from build123d import *

# Parameters (mm, degrees)
F0_W     = 3.81
F0_H     = 16.51
F1_DEPTH = 25.4
F2_W     = 12.7
F2_H     = 5.08
F3_DEPTH = 13.97
F4_R     = 5.08
F6_DEPTH = 25.4
F7_R     = 1.905
F8_DEPTH = 25.4


with BuildPart() as f1:
    # F0 (on Right) → F1 (new body)
    with BuildSketch(Plane.YZ):
        with Locations((-1.905, -8.255)):
            Rectangle(F0_W, F0_H)
    extrude(amount=F1_DEPTH)

    # F2 (on face) → F3 (join)
    with BuildSketch(Plane.XZ.offset(3.81)):
        Polygon((19.05, 0), (12.7, 0), (6.35, 0), (6.35, -5.08), (19.05, -5.08), align=None)
        with Locations((12.7, -13.97)):
            Rectangle(F2_W, F2_H)
    extrude(amount=F3_DEPTH)

    # F4
    f4_edges = [f1.edges().sort_by_distance(p)[0] for p in [
        (19.05, -17.78, -2.54),
        (6.35, -17.78, -2.54),
        (19.05, -17.78, -13.97),
        (6.35, -17.78, -13.97),
    ]]
    fillet(f4_edges, radius=F4_R)

    # F5 (on face) → F6 (cut)
    with BuildSketch(Plane.XY):
        with BuildLine():
            ThreePointArc((15.0495, -11.43), (11.038653, -9.768653), (12.7, -13.7795))
            ThreePointArc((12.7, -13.7795), (14.361347, -13.091347), (15.0495, -11.43))
        make_face()
    extrude(amount=-F6_DEPTH, mode=Mode.SUBTRACT)

    # F7 (on face) → F8 (cut)
    with BuildSketch(Plane.XZ.offset(3.81)):
        with Locations((3.407462, -8.255)):
            Circle(F7_R)
        with Locations((21.952828, -8.255)):
            Circle(F7_R)
    extrude(amount=-F8_DEPTH, mode=Mode.SUBTRACT)


solid = f1.part
The listing builds one solid part. Answer for the finished solid, in the listing's coordinates (mm). A direction names the side the tool comes from. Give positions to 0.01 mm unless a question says otherwise; leave off trailing zeros. Order: outer loops, then holes, each group sorted by start corner. A loop starts at its lowest first (then second) coordinate and runs counter-clockwise, first axis right, second up. Notation, with made-up numbers: (-4.75, -40) - (36.25, -40) arc R25 ccw to (36.25, -9) - close; hole circle Ø6 at (-19, 73.5). An arc over 180 degrees is marked (long way). One line per item, written item: value. Start each with the question number.
1) A cutting plane is placed at A-A on y = -4.5. Give the vertices of the cut face in (x, z).
2) A cutting plane is placed at D-D on x = 22.5. Give the vertices of the cut face in (y, z), then the cut area to 3 significant figures.
3) A cutting plane is placed at C-C on y = -13.25. Give the vertices of the cut face in (x, z).
4) Given pin 1 Ø5 at (x, z) = (11, -8.5) entering from -Y; pin 2 Ø1 at (x, y) = (4.5, -13) entering from -Z; pin 3 Ø1.5 at (y, z) = (-9.5, -13) entering from -X; pin 4 Ø1.5 at (y, z) = (-10, -2) entering from +X, each flat-ended and moving along its own axis, determine where each tip first touches the part or whether it passes through.
5) Find the intervals of material crossed by L1, parallel to X at y = -11.43, z = -3.85; L2, parallel to Z at x = 10.5, y = -6.25, in increasing order.
6) The mould has two halves that part along X. Classify faces 6 (the face through (20.05, -1.93, -8.17)), 7 (the face through (25.4, -2, -8)), 8 (the face through (13, -7, -16.51)): released by +X, released by -X, zero draft, split by the parting line, or undercut.
7) A cutting plane is placed at B-B on z = -1.75. Give the vertices of the cut face in (x, y), then the cut area to 3 significant figures.
8) A tool of negligible diameter and unlimited length cuts with its end or side. For faces 1 (the face through (13, -17.78, -14)), 2 (the face through (19.05, -8, -3)), 3 (the face through (6.35, -8, -14)), 4 (the face through (13, 0, -8)), 5 (the face through (14, -9, -5.08)), from which of +Z, -Z, +X, -X, +Y, -Y can it reach the whole face along a straight path? Write none if from no direction.
Answer sheet:
1. outline: (6.35, -16.51) - (19.05, -16.51) - (19.05, -11.43) - (6.35, -11.43) - close; (6.35, -5.08) - (19.05, -5.08) - (19.05, 0) - (6.35, 0) - close
2. outline: (-3.81, -16.51) - (0, -16.51) - (0, -10.08) - (-3.81, -10.08) - close; (-3.81, -6.43) - (0, -6.43) - (0, 0) - (-3.81, 0) - close
2. area: 49.0 mm2
3. outline: (6.38, -16.51) - (11.21, -16.51) - (11.21, -11.43) - (6.38, -11.43) - close; (6.38, -5.08) - (11.21, -5.08) - (11.21, 0) - (6.38, 0) - close; (14.19, -16.51) - (19.02, -16.51) - (19.02, -11.43) - (14.19, -11.43) - close; (14.19, -5.08) - (19.02, -5.08) - (19.02, 0) - (14.19, 0) - close
4. pin 1: stops at y = -3.81
4. pin 2: passes through
4. pin 3: stops at x = 6.35
4. pin 4: stops at x = 19.05
5. L1: x = 6.35 to 10.35, 15.05 to 19.05
5. L2: z = -16.51 to -11.43, -5.08 to 0
6. face 6: undercut
6. face 7: released by +X
6. face 8: zero draft
7. outline: (0, -3.81) - (6.35, -3.81) - (6.35, -12.7) arc R5.08 ccw to (11.43, -17.78) - (13.97, -17.78) arc R5.08 ccw to (19.05, -12.7) - (19.05, -3.81) - (25.4, -3.81) - (25.4, 0) - (0, 0) - close; hole (12.7, -13.78) arc R2.35 ccw to (15.05, -11.43) arc R2.35 ccw (long way) to start
7. area: 246 mm2
8. face 1: +Z, -Z, +X, -X, -Y
8. face 2: +Z, -Z, +X, -Y
8. face 3: +Z, -Z, -X, -Y
8. face 4: +Z, -Z, +X, -X, +Y
8. face 5: +X, -X, -Y
